The model under review builds one solid part; all positions refer to its coordinate system, in mm. A direction names the side the tool comes from. Round coordinates to 2 decimals unless told otherwise and drop trailing zeros. Loops run counter-clockwise (first coordinate to the right, second up) from the corner with the lowest first, then second, coordinate; pieces in that order, holes last. Notation, with made-up numbers: (-24.5, 79) -> (21.5, 79) arc R23 ccw to (21.5, 107) -> close; hole circle Ø9 at (10.25, 66.25). An arc over 180 degrees is marked (long way). Use a Markdown table: item, result. Add a question column.
1) Mouldability with a two-part tool opening along Y and no side actions: class faces 6 (the flat face through (-11, 23.5, 6)), 7 (the flat face through (12.5, 0, 7)), 8 (the flat face through (-13, 6, 13)) as released by +Y, released by -Y, zero draft, split by the parting line, or undercut.
2) Consider section B-B on x = 10.5. Give the boundary of the cut face in (y, z).
3) Insertion check: pin 1 (4 mm diameter, centred on y = 28.5, z = 4.5, fed in from +X); pin 2 (3 mm diameter, centred on x = 9, z = 8.5, fed in from +Y); pin 3 (1.5 mm diameter, centred on x = 1, y = 18, fed in from -Z). Each pin has a flat end and moves straight along its axis. Give the tip position at first contact, or say it passes through.
4) Consider section C-C on z = 7.5. Give the boundary of the cut face in (x, y), plus the area to 3 significant figures.
5) For faces 1 (the flat face through (10, 23.5, 6)), 2 (the flat face through (-15.5, 0, 6)), 3 (the flat face through (-5.538, 30, 7)), 4 (the flat face through (1.538, 28, 7)), 5 (the flat face through (7, 20.5, 7)), list the 3-axis set-ups (+Z, -Z, +X, -X, +Y, -Y) from which the entire face can be reached by the end or side of a thin tool; tool diameter is ignored.
6) Wall thickness on probe 1 along X at (y, z) = (13.5, 2); probe 2 along Y at (x, z) = (-8.5, 1.5); probe 3 along Y at (x, z) = (-3, 3): over which ranges is each line inside the solid? List them lowest first.
7) Consider section A-A on y = 7.5. Give the boundary of the cut face in (x, z).
from build123d import *

# Parameters (mm, degrees)
CROQUIS1_W              = 31
CROQUIS1_H              = 47
SALIENTE_EXTRUIR1_DEPTH = 13
CROQUIS2_W              = 25
CROQUIS2_H              = 41
CORTAR_EXTRUIR1_DEPTH   = 13
CROQUIS3_W              = 3.075448652
CROQUIS3_H              = 33.686173061
CORTAR_EXTRUIR2_DEPTH   = 13
CROQUIS4_W              = 4
CROQUIS4_H              = 13
SALIENTE_EXTRUIR2_DEPTH = 13


with BuildPart() as part:
    # Croquis1 → Saliente-Extruir1 (new body)
    with BuildSketch(Plane.XY):
        Rectangle(CROQUIS1_W, CROQUIS1_H)
    extrude(amount=SALIENTE_EXTRUIR1_DEPTH)

    # Croquis2 → Cortar-Extruir1 (cut)
    with BuildSketch(Plane.XY.offset(13)):
        Rectangle(CROQUIS2_W, CROQUIS2_H)
    extrude(amount=-CORTAR_EXTRUIR1_DEPTH, mode=Mode.SUBTRACT)

    # Croquis3 → Cortar-Extruir2 (cut)
    with BuildSketch(Plane(origin=(0, 23.5, 0), x_dir=(1, 0, 0), z_dir=(0, 1, 0))):
        with Locations((0, -5.988894029)):
            Rectangle(CROQUIS3_W, CROQUIS3_H)
    extrude(amount=-CORTAR_EXTRUIR2_DEPTH, mode=Mode.SUBTRACT)

    # Croquis4 → Saliente-Extruir2 (add)
    with BuildSketch(Plane(origin=(0, 23.5, 0), x_dir=(1, 0, 0), z_dir=(0, 1, 0))):
        with Locations((3.537724326, -6.5)):
            Rectangle(CROQUIS4_W, CROQUIS4_H)
        with Locations((-3.537724326, -6.5)):
            Rectangle(CROQUIS4_W, CROQUIS4_H)
    extrude(amount=SALIENTE_EXTRUIR2_DEPTH)


solid = part.part
Result set:
| question | item | result |
|---|---|---|
| 1 | face 6 | released by +Y |
| 1 | face 7 | undercut |
| 1 | face 8 | zero draft |
| 2 | outline | (-23.5, 0) -> (-20.5, 0) -> (-20.5, 13) -> (-23.5, 13) -> close; (20.5, 0) -> (23.5, 0) -> (23.5, 13) -> (20.5, 13) -> close |
| 3 | pin 1 | x = 5.54 |
| 3 | pin 2 | y = 23.5 |
| 3 | pin 3 | through |
| 4 | outline | (-15.5, -23.5) -> (15.5, -23.5) -> (15.5, 23.5) -> (5.54, 23.5) -> (5.54, 36.5) -> (1.54, 36.5) -> (1.54, 20.5) -> (12.5, 20.5) -> (12.5, -20.5) -> (-12.5, -20.5) -> (-12.5, 20.5) -> (-1.54, 20.5) -> (-1.54, 36.5) -> (-5.54, 36.5) -> (-5.54, 23.5) -> (-15.5, 23.5) -> close |
| 4 | area | 527 mm2 |
| 5 | face 1 | +Z, -Z, +X, +Y |
| 5 | face 2 | +Z, -Z, -X, +Y, -Y |
| 5 | face 3 | +Z, -Z, -X, +Y |
| 5 | face 4 | +Z, -Z, +Y |
| 5 | face 5 | +Z, -Z |
| 6 | probe 1 | -15.5 to -12.5, 12.5 to 15.5 |
| 6 | probe 2 | -23.5 to -20.5, 20.5 to 23.5 |
| 6 | probe 3 | -23.5 to -20.5, 20.5 to 36.5 |
| 7 | outline | (-15.5, 0) -> (-12.5, 0) -> (-12.5, 13) -> (-15.5, 13) -> close; (12.5, 0) -> (15.5, 0) -> (15.5, 13) -> (12.5, 13) -> close |
